```python
from build123d import *

# Parameters (mm, degrees)
SKETCH2_W               = 9.652
SKETCH2_H               = 3.048
SKETCH2_W_2             = 3.048
SKETCH2_H_2             = 35.052
BOSS_EXTRUDE1_DEPTH     = 315
SKETCH3_W               = 25.4
SKETCH3_H               = 76.2
SKETCH3_W_2             = 19.304
SKETCH3_H_2             = 70.104
BOSS_EXTRUDE2_DEPTH     = 50
CUT_EXTRUDE1_DEPTH      = 1
CUT_EXTRUDE1_DEPTH_BACK = 77.2


with BuildPart() as part:
    # Sketch2 → Boss-Extrude1 (new body)
    with BuildSketch(Plane.XY):
        Polygon((-12.7, 0), (-9.652, 0), (-9.652, 35.052), (-9.652, 38.1), (-12.7, 38.1), align=None)
        with Locations((-4.826, 36.576)):
            Rectangle(SKETCH2_W, SKETCH2_H)
        Polygon((0, 38.1), (0, 35.052), (9.652, 35.052), (9.652, 0), (12.7, 0), (12.7, 38.1), align=None)
        with Locations((11.176, -17.526)):
            Rectangle(SKETCH2_W_2, SKETCH2_H_2)
        Polygon((-9.652, -35.052), (-9.652, 0), (-12.7, 0), (-12.7, -38.1), (0, -38.1), (0, -35.052), align=None)
        Polygon((9.652, -35.052), (0, -35.052), (0, -38.1), (12.7, -38.1), (12.7, -35.052), align=None)
    extrude(amount=BOSS_EXTRUDE1_DEPTH)

    # Sketch3 → Boss-Extrude2 (add)
    with BuildSketch(Plane(origin=(0, 0, 0), x_dir=(-1, 0, 0), z_dir=(0, 0, -1))):
        Rectangle(SKETCH3_W, SKETCH3_H)
        Rectangle(SKETCH3_W_2, SKETCH3_H_2, mode=Mode.SUBTRACT)
    extrude(amount=BOSS_EXTRUDE2_DEPTH)

    # Sketch4 → Cut-Extrude1 (cut, two sides)
    with BuildSketch(Plane(origin=(0, 38.1, 0), x_dir=(1, 0, 0), z_dir=(0, 1, 0))) as cut_extrude1_sk:
        Polygon((-12.7, 46.179632344), (-70.94979307, -6.803292614), (-12.7, -1.217788135), align=None)
        Polygon((-77.560178635, 62.134722349), (-70.94979307, -6.803292614), (-12.7, 46.179632344), (-12.7, 50), (12.7, 50), (12.7, 1.217788135), (70.94979307, 6.803292614), (64.339407504, 75.741307577), align=None)
        Polygon((-12.7, 46.179632344), (-12.7, -1.217788135), (0, 0), (-9.501519639, 49.088910403), align=None)
        Polygon((-12.7, 50), (-12.7, 46.179632344), (-9.501519639, 49.088910403), (0, 0), (12.7, 1.217788135), (12.7, 50), align=None)
    extrude(amount=CUT_EXTRUDE1_DEPTH, mode=Mode.SUBTRACT)
    extrude(cut_extrude1_sk.sketch, amount=-CUT_EXTRUDE1_DEPTH_BACK, mode=Mode.SUBTRACT)


solid = part.part
```
Can you work these out from the model? Positions are in its coordinate system, mm. A direction names the side the tool comes from. Round coordinates to 2 decimals unless told otherwise and drop trailing zeros. Loops run counter-clockwise (first coordinate to the right, second up) from the corner with the lowest first, then second, coordinate; pieces in that order, holes last.
Item 1: Which directions (+Z, -Z, +X, -X, +Y, -Y) give clear straight access to the entire face, cutting with the end or side of a thin tool? Please do faces 5 (the flat face through (0, 38.1, 159)), 6 (the flat face through (9.652, 0, 159)).
Item 2: Suppose I cut it at B-B, the plane y = 31. Write out the boundary of the cut face in (x, z), then the cut area to 3 significant figures.
Item 3: Suppose I cut it at A-A, the plane z = 52. Write out the boundary of the cut face in (x, y), then the cut area to 3 significant figures.
Item 4: If we mould it in two halves opening along X, with no side actions, what happens to faces 1 (the flat face through (0, -38.1, 159)), 2 (the flat face through (12.7, -1, 159)), 3 (the flat face through (0, 35.052, 159)), 4 (the flat face through (-12.7, -1, 160))? For each: +X half, -X half, draft (parallel to the pull), parting line (faces both ways), or undercut.
Item 5: Suppose I cut it at C-C, the plane x = 0. Write out the boundary of the cut face in (y, z), then the cut area to 3 significant figures.
Item 6: Please list where these lines run through material, in increasing order: L1, parallel to X at y = 21, z = 146.5; L2, parallel to Y at x = 4.75, z = 141; L3, parallel to Z at x = -11.5, y = -17.5.
Item 7: Will this pin go through, and if not, where does the flat tip stop? pin 1 Ø6 at (x, y) = (4.5, 11.5) entering from +Z.
Reported:
1. face 5: +Z, -Z, +X, -X, +Y
1. face 6: +Z, -Z
2. outline: (-12.7, 1.22) - (-9.65, 0.93) - (-9.65, 315) - (-12.7, 315) - close; (9.65, -0.93) - (12.7, -1.22) - (12.7, 315) - (9.65, 315) - close
2. area: 1,920 mm2
3. outline: (-12.7, -38.1) - (12.7, -38.1) - (12.7, 38.1) - (-12.7, 38.1) - close; hole (-9.65, -35.05) - (9.65, -35.05) - (9.65, 35.05) - (-9.65, 35.05) - close
3. area: 582 mm2
4. face 1: draft
4. face 2: +X half
4. face 3: undercut
4. face 4: -X half
5. outline: (-38.1, 0) - (-35.05, 0) - (-35.05, 315) - (-38.1, 315) - close; (35.05, 0) - (38.1, 0) - (38.1, 315) - (35.05, 315) - close
5. area: 1,920 mm2
6. L1: x = -12.7 to -9.65, 9.65 to 12.7
6. L2: y = -38.1 to -35.05, 35.05 to 38.1
6. L3: z = 1.1 to 315
7. pin 1: passes through
